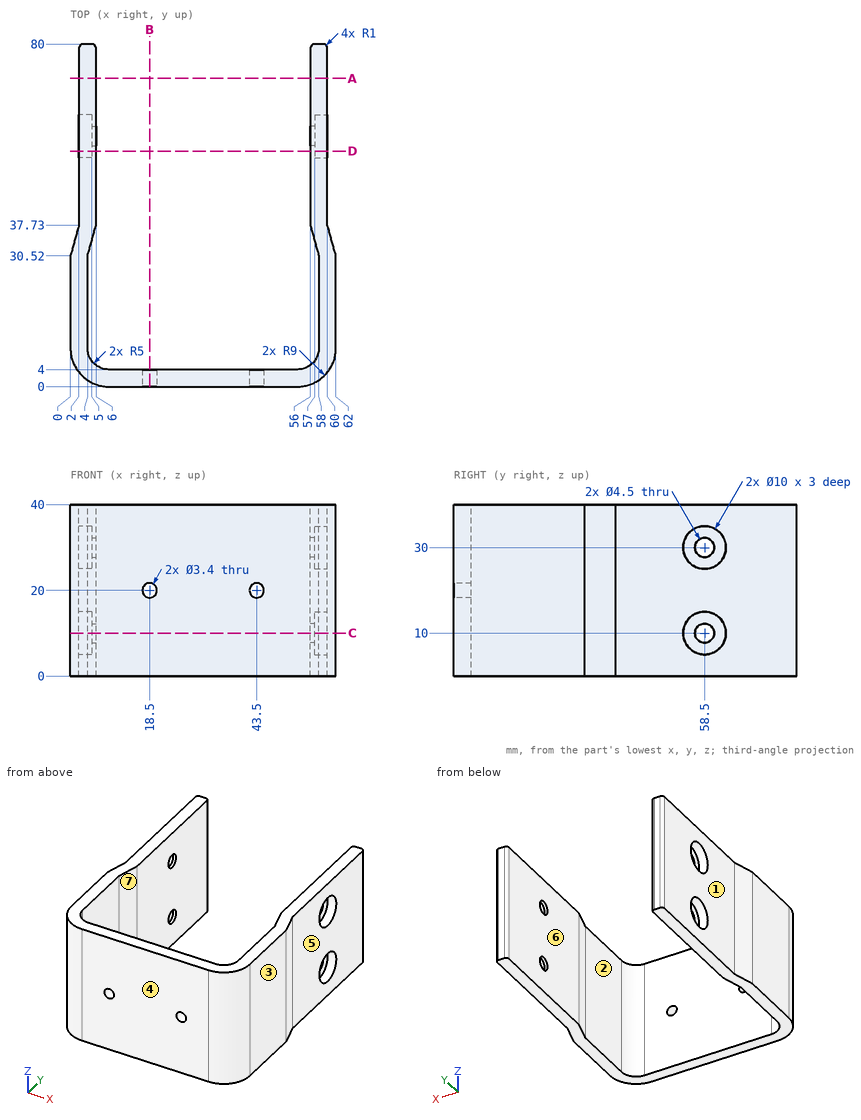
Here's the drawing with two shaded views (mm, measured from the low corner). I have some questions. A direction names the side the tool comes from. Round coordinates to 2 decimals unless told otherwise and drop trailing zeros. Order: outer loops, then holes, each group sorted by start corner. A loop starts at its lowest first (then second) coordinate and runs counter-clockwise, first axis right, second up. Notation, with made-up numbers: M 23,42.25 L 38,42.25 A7 cw 38,46.25 Z; hole C 39,83.25 d4. An arc over 180 degrees is marked long. Answer in a Markdown table with one row per item.
Item 1: If I drill on L1, parallel to X at y = 45, z = 28.5; L2, parallel to Z at x = 18.5, y = 1.55; L3, parallel to X at y = 62, z = 30.5, over which ranges is the centre line in solid material (lowest first)? Write a range as from..to.
A:
| item | result |
|---|---|
| L1 | x = 2..6, 56..60 |
| L2 | z = 0..18.3, 21.7..40 |
| L3 | x = 5..6, 56..57 |
Item 2: Imagine slicing it at D-D, the plane y = 55. Write out the boundary of the cut face in (x, z).
A:
| item | result |
|---|---|
| outline | M 2,0 L 6,0 L 6,40 L 2,40 L 2,33.57 L 5,33.57 L 5,26.43 L 2,26.43 L 2,13.57 L 5,13.57 L 5,6.43 L 2,6.43 Z; M 56,0 L 60,0 L 60,6.43 L 57,6.43 L 57,13.57 L 60,13.57 L 60,26.43 L 57,26.43 L 57,33.57 L 60,33.57 L 60,40 L 56,40 Z |
Item 3: Imagine slicing it at B-B, the plane x = 18.5. Write out the boundary of the cut face in (y, z).
A:
| item | result |
|---|---|
| outline | M 0,0 L 4,0 L 4,18.3 L 0,18.3 Z; M 0,21.7 L 4,21.7 L 4,40 L 0,40 Z |
Item 4: Thinking about a two-plate mould opening in X: for the marked faces 1, 2, 3 and 4, which applies, +X half, -X half, draft (parallel to the pull), parting line (faces both ways), or undercut?
A:
| item | result |
|---|---|
| face 1 | -X half |
| face 2 | undercut |
| face 3 | +X half |
| face 4 | draft |
Item 5: For the marked faces 5, 6 and 7, which set-ups out of +Z, -Z, +X, -X, +Y, -Y let a thin tool reach every point of the face, with its end or its side?
A:
| item | result |
|---|---|
| face 5 | +Z, -Z, +X, +Y |
| face 6 | +Z, -Z, +Y |
| face 7 | +Z, -Z |
Item 6: Imagine slicing it at A-A, the plane y = 72. Write out the boundary of the cut face in (x, z), and give its area (3 significant figures).
A:
| item | result |
|---|---|
| outline | M 2,0 L 6,0 L 6,40 L 2,40 Z; M 56,0 L 60,0 L 60,40 L 56,40 Z |
| area | 320 mm2 |
Item 7: I'm going to push flat-ended pins straight in: pin 1 (8 mm diameter, centred on x = 27.5, z = 19.5, fed in from +Y); pin 2 (5 mm diameter, centred on y = 58, z = 30.5, fed in from -X); pin 3 (13 mm diameter, centred on y = 58.5, z = 30, fed in from +X); pin 4 (10 mm diameter, centred on x = 48.5, y = 62, fed in from +Z). Where does each tip first touch, or does it pass through?
A:
| item | result |
|---|---|
| pin 1 | stops at y = 4 |
| pin 2 | stops at x = 5 |
| pin 3 | stops at x = 60 |
| pin 4 | passes through |
Item 8: Imagine slicing it at C-C, the plane z = 10. State how many separate pieces and enclosed holes the cut face has, and give its area (3 significant figures).
A:
| item | result |
|---|---|
| separate pieces | 3 |
| enclosed holes | 0 |
| area | 762 mm2 |
